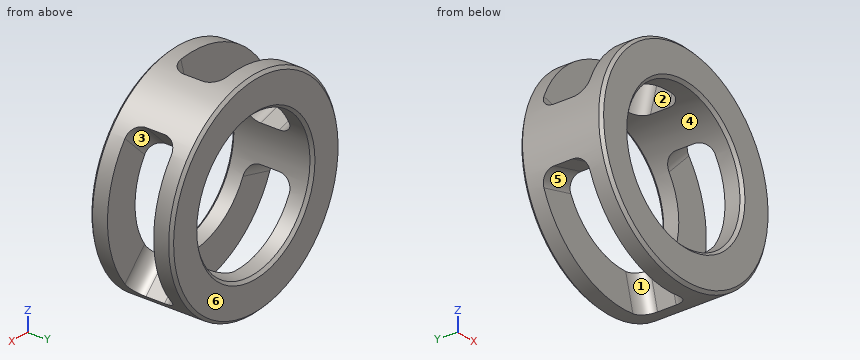
```python
from build123d import *

# Parameters (mm, degrees)
SKETCH1_R           = 11.5
SKETCH1_R_2         = 7.75
BOSS_EXTRUDE1_DEPTH = 4.42
CUT_EXTRUDE1_DEPTH  = 2.5
FILLET1_R           = 1.5
CHAMFER1_SIZE       = 0.3


with BuildPart() as part:
    # Sketch1 → Boss-Extrude1 (new, symmetric)
    with BuildSketch(Plane(origin=(0, 0, 0), x_dir=(1, 0, 0), z_dir=(0, 1, 0))):
        with Locations(Location((0, 0, 0), (0, 0, 270))):
            Circle(SKETCH1_R)
        with Locations(Location((0, 0, 0), (0, 0, 270))):
            Circle(SKETCH1_R_2, mode=Mode.SUBTRACT)
    extrude(amount=BOSS_EXTRUDE1_DEPTH, both=True)

    # Sketch2 → Cut-Extrude1 (cut, symmetric)
    with BuildSketch(Plane(origin=(0, 0, 0), x_dir=(1, 0, 0), z_dir=(0, 1, 0))):
        with BuildLine():
            Line((4.772970773, 4.772970773), (8.838834765, 8.838834765))
            ThreePointArc((8.838834765, 8.838834765), (12.5, 0), (8.838834765, -8.838834765))
            Line((8.838834765, -8.838834765), (4.772970773, -4.772970773))
            ThreePointArc((4.772970773, -4.772970773), (6.75, 0), (4.772970773, 4.772970773))
        make_face()
        with BuildLine():
            Line((1.747028554, -6.519999327), (3.235238064, -12.074072829))
            ThreePointArc((3.235238064, -12.074072829), (-6.25, -10.825317547), (-12.074072829, -3.235238064))
            Line((-12.074072829, -3.235238064), (-6.519999327, -1.747028554))
            ThreePointArc((-6.519999327, -1.747028554), (-3.375, -5.845671476), (1.747028554, -6.519999327))
        make_face()
        with BuildLine():
            Line((-6.519999327, 1.747028554), (-12.074072829, 3.235238064))
            ThreePointArc((-12.074072829, 3.235238064), (-6.25, 10.825317547), (3.235238064, 12.074072829))
            Line((3.235238064, 12.074072829), (1.747028554, 6.519999327))
            ThreePointArc((1.747028554, 6.519999327), (-3.375, 5.845671476), (-6.519999327, 1.747028554))
        make_face()
    extrude(amount=CUT_EXTRUDE1_DEPTH, both=True, mode=Mode.SUBTRACT)

    # Fillet1
    fillet1_edges = [part.edges().sort_by_distance(p)[0] for p in [
        (6.805902769, -2.5, -6.805902769),
        (6.805902769, -2.5, 6.805902769),
        (6.805902769, 2.5, -6.805902769),
        (6.805902769, 2.5, 6.805902769),
        (2.491133309, -2.5, 9.297036078),
        (-9.297036078, -2.5, 2.491133309),
        (2.491133309, 2.5, 9.297036078),
        (-9.297036078, 2.5, 2.491133309),
        (-9.297036078, -2.5, -2.491133309),
        (2.491133309, -2.5, -9.297036078),
        (-9.297036078, 2.5, -2.491133309),
        (2.491133309, 2.5, -9.297036078),
    ]]
    fillet(fillet1_edges, radius=FILLET1_R)

    # Chamfer1
    chamfer1_edges = [part.edges().sort_by_distance(p)[0] for p in [
        (0, -4.42, -11.5),
        (0, 4.42, -11.5),
        (0, -4.42, -7.75),
        (0, 4.42, -7.75),
    ]]
    chamfer(chamfer1_edges, length=CHAMFER1_SIZE)


solid = part.part
```
Could you check a few things on this model? Use its own coordinates, in mm. Face numbers are marked on the shaded views. A direction names the side the tool comes from. Give positions to 0.01 mm unless a question says otherwise; leave off trailing zeros. Order: outer loops, then holes, each group sorted by start corner. A loop starts at its lowest first (then second) coordinate and runs counter-clockwise, first axis right, second up.
Q1. Suppose I cut it at D-D, the plane y = 2. Write out the boundary of the cut face in (x, z).
Q2. I'm going to push flat-ended pins straight in: P1, Ø2, axis at y = 3, z = 7.5, coming from the -X side; P2, Ø5, axis at y = -1.5, z = -7.5, coming from the -X side. Where does each tip first touch, or does it pass through?
Q3. Suppose I cut it at C-C, the plane y = -0.25. Write out the boundary of the cut face in (x, z).
Q4. Suppose I cut it at B-B, the plane z = 0. Write out the boundary of the cut face in (x, y).
Q5. For the marked faces 1, 2 and 3, which set-ups out of +Z, -Z, +X, -X, +Y, -Y let a thin tool reach every point of the face, with its end or its side?
Q6. If I drill on line 1 along Y through (x, z) = (0.75, 9.75); line 2 along X through (y, z) = (0, 0); line 3 along Z through (x, y) = (-4.5, 3.75), over which ranges is the centre line in solid material (lowest first)?
Q7. We'd pull the mould along X, two halves only. Please class the marked faces 4, 5 and 6: +X half, -X half, draft (parallel to the pull), parting line (faces both ways), or undercut.
Q8. Suppose I cut it at A-A, the plane x = 0. Write out the boundary of the cut face in (y, z).
Solution:
1. outline: (-11, -3.34) - (-7.38, -2.37) arc R7.75 cw to (-7.38, 2.37) - (-11, 3.34) arc R11.5 ccw to start; (1.63, -7.58) - (2.61, -11.2) arc R11.5 ccw to (8.4, -7.86) - (5.74, -5.2) arc R7.75 cw to start; (1.63, 7.58) arc R7.75 cw to (5.74, 5.2) - (8.4, 7.86) arc R11.5 ccw to (2.61, 11.2) - close
2. P1: stops at x = -9.49
2. P2: stops at x = -10.25
3. outline: (-11.11, -2.98) - (-7.49, -2.01) arc R7.75 cw to (-7.49, 2.01) - (-11.11, 2.98) arc R11.5 ccw to start; (2.01, -7.49) - (2.98, -11.11) arc R11.5 ccw to (8.13, -8.13) - (5.48, -5.48) arc R7.75 cw to start; (2.01, 7.49) arc R7.75 cw to (5.48, 5.48) - (8.13, 8.13) arc R11.5 ccw to (2.98, 11.11) - close
4. outline: (-11.5, -4.12) - (-11.2, -4.42) - (-8.05, -4.42) - (-7.75, -4.12) - (-7.75, 4.12) - (-8.05, 4.42) - (-11.2, 4.42) - (-11.5, 4.12) - close; (7.75, -4.12) - (8.05, -4.42) - (11.2, -4.42) - (11.5, -4.12) - (11.5, -2.5) - (7.75, -2.5) - close; (7.75, 2.5) - (11.5, 2.5) - (11.5, 4.12) - (11.2, 4.42) - (8.05, 4.42) - (7.75, 4.12) - close
5. face 1: -Z, -X
5. face 2: +Z, -X
5. face 3: +X
6. line 1: y = -4.42 to -2.5, 2.5 to 4.42
6. line 2: x = -11.5 to -7.75
6. line 3: z = -10.58 to -6.31, 6.31 to 10.58
7. face 4: undercut
7. face 5: +X half
7. face 6: draft
8. outline: (-4.42, -11.2) - (-4.12, -11.5) - (-2.5, -11.5) - (-2.5, -7.75) - (-4.12, -7.75) - (-4.42, -8.05) - close; (-4.42, 8.05) - (-4.12, 7.75) - (-2.5, 7.75) - (-2.5, 11.5) - (-4.12, 11.5) - (-4.42, 11.2) - close; (2.5, -11.5) - (4.12, -11.5) - (4.42, -11.2) - (4.42, -8.05) - (4.12, -7.75) - (2.5, -7.75) - close; (2.5, 7.75) - (4.12, 7.75) - (4.42, 8.05) - (4.42, 11.2) - (4.12, 11.5) - (2.5, 11.5) - close
